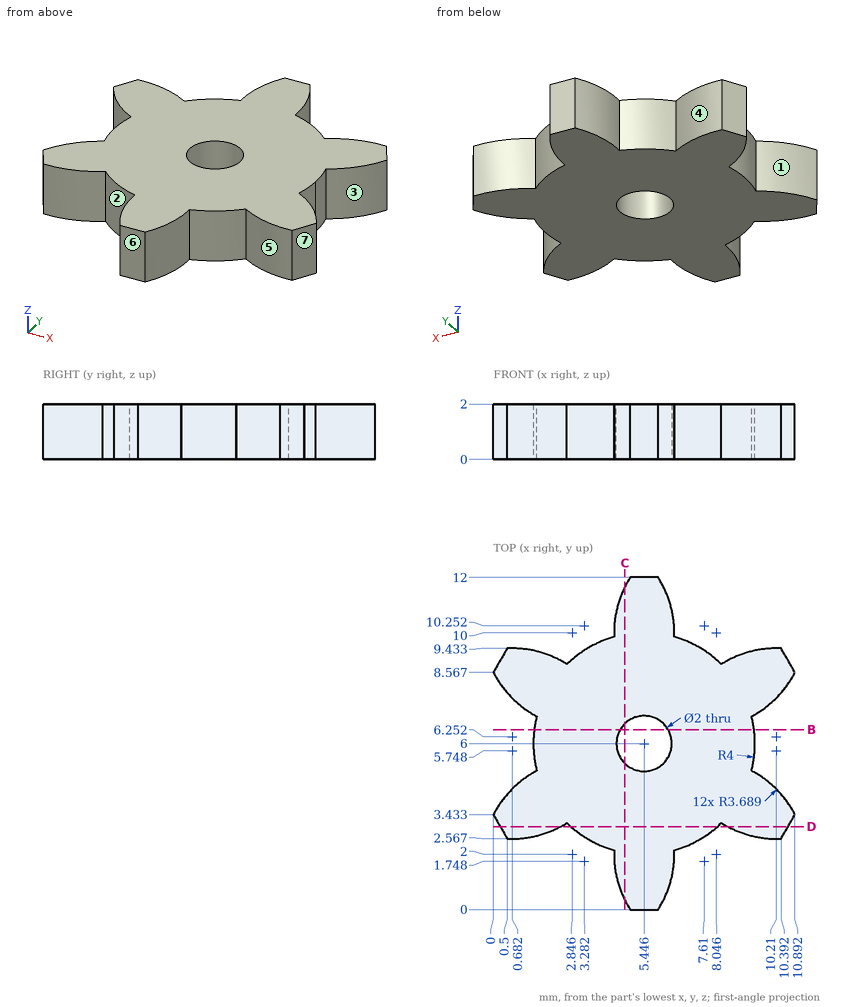
Here's the drawing with two shaded views (mm, measured from the low corner). I have some questions. A direction names the side the tool comes from. Round coordinates to 2 decimals unless told otherwise and drop trailing zeros. Loops run counter-clockwise (first coordinate to the right, second up) from the corner with the lowest first, then second, coordinate; pieces in that order, holes last. Notation, with made-up numbers: (29.5, 19.5) -> (85.5, 19.5) arc R22 cw to (85.5, 37.5) -> close; hole circle Ø1 at (34, 86.25). An arc over 180 degrees is marked (long way). Answer as CSV lines item,"result". Start each with the question number.
1. I'm going to push a flat-ended pin straight in: P1, Ø1.8, axis at x = 5.45, y = 6, coming from the +Z side. Where does the tip first touch, or does it pass through?
2. Imagine slicing it at D-D on y = 3. State how many separate pieces and enclosed holes the cut face has, plus the area to 3 significant figures.
3. If we mould it in two halves opening along X, with no side actions, what happens to the marked faces 5, 6 and 7? For each: pulls with the +X half, pulls with the -X half, needs draft (parallel to the pull), parting line crosses it, or undercut.
4. I need wall thicknesses on probe 1 along Y at (x, z) = (5.75, 1.3); probe 2 along Y at (x, z) = (5, 1.5) (1 decimal); probe 3 along X at (y, z) = (4, 0.25). Which ranges of each line are inside material? Lowest first, please. Write a range as from..to.
5. Imagine slicing it at C-C on x = 4.75. Write out the boundary of the cut face in (y, z).
6. Imagine slicing it at B-B on y = 6.5. Write out the boundary of the cut face in (x, z) (1 decimal), plus the area to 3 significant figures.
7. For the marked faces 1, 2, 3 and 4, which set-ups out of +Z, -Z, +X, -X, +Y, -Y let a thin tool reach every point of the face, with its end or its side?
Solution:
1,P1,"through"
2,separate pieces,"3"
2,enclosed holes,"0"
2,area,"19.3 mm²"
3,face 5,"undercut"
3,face 6,"needs draft"
3,face 7,"pulls with the +X half"
4,probe 1,"0..5.05, 6.95..12"
4,probe 2,"0..5.1, 6.9..12"
4,probe 3,"0.36..10.53"
5,outline,"(0.34, 0) -> (5.28, 0) -> (5.28, 2) -> (0.34, 2) -> close; (6.72, 0) -> (11.66, 0) -> (11.66, 2) -> (6.72, 2) -> close"
6,outline,"(1.5, 0) -> (4.6, 0) -> (4.6, 2) -> (1.5, 2) -> close; (6.3, 0) -> (9.4, 0) -> (9.4, 2) -> (6.3, 2) -> close"
6,area,"12.4 mm²"
7,face 1,"+Z, -Z, -X"
7,face 2,"+Z, -Z, -Y"
7,face 3,"+Z, -Z, +X"
7,face 4,"+Z, -Z, +Y"
